For this review, take the finished solid that the model builds, in its own axes (mm). A direction names the side the tool comes from. Give positions to 0.01 mm unless a question says otherwise; leave off trailing zeros. Loops run counter-clockwise (first coordinate to the right, second up) from the corner with the lowest first, then second, coordinate; pieces in that order, holes last. Notation, with made-up numbers: (25.25, 71) - (52.25, 71) arc R10 cw to (52.25, 81) - close; hole circle Ø9 at (40, 21.25). An arc over 180 degrees is marked (long way). Answer as CSV lines item,"result".
from build123d import *

# Parameters (mm, degrees)
BOSS_EXTRUDE1_DEPTH          = 38.1
FILLET1_R                    = 5.08
FILLET2_R                    = 5.08
SHELL1_T                     = -2.54
F_97_0_0059_DIAMETER_HOLE1_D = 6.35
F_1_4_0_25_DIAMETER_HOLE1_D  = 6.35


with BuildPart() as part:
    # Sketch1 → Boss-Extrude1 (new body)
    with BuildSketch(Plane.XY):
        Polygon((0, 0), (0, 69.85), (44.45, 69.85), (44.45, 44.45), (101.6, 44.45), (101.6, 0), align=None)
    extrude(amount=BOSS_EXTRUDE1_DEPTH)

    # Fillet1
    fillet1_edges = [part.edges().sort_by_distance(p)[0] for p in [
        (0, 0, 19.05),
        (0, 69.85, 19.05),
        (44.45, 69.85, 19.05),
        (44.45, 44.45, 19.05),
        (101.6, 44.45, 19.05),
        (101.6, 0, 19.05),
    ]]
    fillet(fillet1_edges, radius=FILLET1_R)

    # Fillet2
    fillet2_edges = [part.edges().sort_by_distance(p)[0] for p in [
        (101.6, 22.225, 38.1),
        (50.8, 0, 38.1),
        (73.025, 44.45, 38.1),
        (44.45, 57.15, 38.1),
        (22.225, 69.85, 38.1),
        (0, 34.925, 38.1),
        (42.962102448, 68.362102448, 38.1),
        (1.487897552, 68.362102448, 38.1),
        (1.487897552, 1.487897552, 38.1),
        (100.112102448, 42.962102448, 38.1),
        (100.112102448, 1.487897552, 38.1),
        (45.937897552, 45.937897552, 38.1),
    ]]
    fillet(fillet2_edges, radius=FILLET2_R)

    # Shell1
    shell1_openings = [part.faces().sort_by_distance(p)[0] for p in [
        (48.683333333, 38.1, 0),
    ]]
    offset(amount=SHELL1_T, openings=shell1_openings, kind=Kind.INTERSECTION)

    # #97 (0.0059) Diameter Hole1 (through all)
    with Locations(Plane.XY.offset(38.1)):
        with Locations((87.63, 30.48)):
            Hole(F_97_0_0059_DIAMETER_HOLE1_D / 2)

    # 1/4 (0.25) Diameter Hole1 (through all)
    with Locations(Plane.XY.offset(38.1)):
        with Locations((87.63, 13.97), (13.97, 13.97)):
            Hole(F_1_4_0_25_DIAMETER_HOLE1_D / 2)


solid = part.part
1) Insertion check: P1, Ø8, axis at x = 46, z = 17.5, coming from the +Y side; P2, Ø16.5, axis at x = 63.5, z = 17.5, coming from the +Y side; P3, Ø17, axis at y = 56.5, z = 21, coming from the +X side. Each pin has a flat end and moves straight along its axis. Give the tip position at first contact, or say it passes through.
From the geometry:
P1,"stops at y = 69.12"
P2,"stops at y = 44.45"
P3,"stops at x = 44.69"
2) Wall thickness on line 1 (X direction, y = 51, z = 3.5); line 2 (X direction, y = 16.5, z = 25.5); line 3 (X direction, y = 13, z = 37): over which ranges is each line inside the solid? List them lowest first. Write a range as from..to.
From the geometry:
line 1,"x = 0..2.54, 41.91..44.45"
line 2,"x = 0..2.54, 99.06..101.6"
line 3,"x = 1.92..10.95, 16.99..84.61, 90.65..99.68"
3) Consider section A-A on x = 87.63. Write out the cut boundary in (y, z) (3 decimals).
From the geometry:
outline,"(0, 0) - (2.54, 0) - (2.54, 33.02) arc R2.54 cw to (5.08, 35.56) - (10.795, 35.56) - (10.795, 38.1) - (5.08, 38.1) arc R5.08 ccw to (0, 33.02) - close; (17.145, 35.56) - (27.305, 35.56) - (27.305, 38.1) - (17.145, 38.1) - close; (33.655, 35.56) - (39.37, 35.56) arc R2.54 cw to (41.91, 33.02) - (41.91, 0) - (44.45, 0) - (44.45, 33.02) arc R5.08 ccw to (39.37, 38.1) - (33.655, 38.1) - close"
4) Consider section D-D on y = 30.48. Write out the cut boundary in (x, z) (3 decimals).
From the geometry:
outline,"(0, 0) - (2.54, 0) - (2.54, 33.02) arc R2.54 cw to (5.08, 35.56) - (84.455, 35.56) - (84.455, 38.1) - (5.08, 38.1) arc R5.08 ccw to (0, 33.02) - close; (90.805, 35.56) - (96.52, 35.56) arc R2.54 cw to (99.06, 33.02) - (99.06, 0) - (101.6, 0) - (101.6, 33.02) arc R5.08 ccw to (96.52, 38.1) - (90.805, 38.1) - close"
5) Draft analysis for pull direction Y (two halves, no side actions). For faces 6 (the flat face through (73, 41.91, 16)), 7 (the cylindrical face through (100.072, 43.001, 16.741)), 8 (the flat face through (47, 43, 0)), state which applies: pulls with the +Y half, pulls with the -Y half, needs draft (parallel to the pull), parting line crosses it, or undercut.
From the geometry:
face 6,"undercut"
face 7,"pulls with the +Y half"
face 8,"needs draft"
6) Machinability: for faces 1 (the flat face through (44.45, 57, 16)), 2 (the cylindrical face through (84.6, 14.92, 36.81)), 3 (the cylindrical face through (73.354, 42.922, 36.651)), 4 (the cylindrical face through (3.264, 66.546, 16.741)), 5 (the cylindrical face through (100.151, 1.528, 16.741)), which of the approach directions +Z, -Z, +X, -X, +Y, -Y give a long, thin tool a straight path to every point of the face, cutting with its end or side? Answer none if there is none.
From the geometry:
face 1,"+Z, -Z, +X, +Y"
face 2,"+Z, -Z"
face 3,"+Z, +X, +Y"
face 4,"-Z"
face 5,"+Z, -Z, +X, -Y"
7) Consider section B-B on z = 11.5. Write out the cut boundary in (x, y).
From the geometry:
outline,"(0, 5.08) arc R5.08 ccw to (5.08, 0) - (96.52, 0) arc R5.08 ccw to (101.6, 5.08) - (101.6, 39.37) arc R5.08 ccw to (96.52, 44.45) - (49.53, 44.45) arc R5.08 cw to (44.45, 49.53) - (44.45, 64.77) arc R5.08 ccw to (39.37, 69.85) - (5.08, 69.85) arc R5.08 ccw to (0, 64.77) - close; hole (2.54, 5.08) arc R2.54 ccw to (5.08, 2.54) - (96.52, 2.54) arc R2.54 ccw to (99.06, 5.08) - (99.06, 39.37) arc R2.54 ccw to (96.52, 41.91) - (49.53, 41.91) arc R7.62 cw to (41.91, 49.53) - (41.91, 64.77) arc R2.54 ccw to (39.37, 67.31) - (5.08, 67.31) arc R2.54 ccw to (2.54, 64.77) - close"
8) Consider section C-C on y = 13.97. Write out the cut boundary in (x, z) (3 decimals).
From the geometry:
outline,"(0, 0) - (2.54, 0) - (2.54, 33.02) arc R2.54 cw to (5.08, 35.56) - (10.795, 35.56) - (10.795, 38.1) - (5.08, 38.1) arc R5.08 ccw to (0, 33.02) - close; (17.145, 35.56) - (84.455, 35.56) - (84.455, 38.1) - (17.145, 38.1) - close; (90.805, 35.56) - (96.52, 35.56) arc R2.54 cw to (99.06, 33.02) - (99.06, 0) - (101.6, 0) - (101.6, 33.02) arc R5.08 ccw to (96.52, 38.1) - (90.805, 38.1) - close"
